```python
from build123d import *

# Parameters (mm, degrees)
SKETCH1_W                = 18
SKETCH1_H                = 10
BOSS_EXTRUDE1_DEPTH      = 10
SKETCH2_W                = 3
SKETCH2_H                = 5.5
BOSS_EXTRUDE2_DEPTH      = 4
SKETCH3_W                = 3
SKETCH3_H                = 5.5
BOSS_EXTRUDE3_DEPTH      = 4
F_4_0_4_DIAMETER_HOLE1_D = 4


with BuildPart() as part:
    # Sketch1 → Boss-Extrude1 (new body)
    with BuildSketch(Plane.XZ.offset(5)):
        with Locations((-1.5, 5)):
            Rectangle(SKETCH1_W, SKETCH1_H)
    extrude(amount=-BOSS_EXTRUDE1_DEPTH)

    # Sketch2 → Boss-Extrude2 (add)
    with BuildSketch(Plane(origin=(0, 5, 0), x_dir=(-1, 0, 0), z_dir=(0, 1, 0))):
        with Locations((-6, 2.75)):
            Rectangle(SKETCH2_W, SKETCH2_H)
    extrude(amount=BOSS_EXTRUDE2_DEPTH)

    # Sketch3 → Boss-Extrude3 (add)
    with BuildSketch(Plane.XZ.offset(5)):
        with Locations((6, 2.75)):
            Rectangle(SKETCH3_W, SKETCH3_H)
    extrude(amount=BOSS_EXTRUDE3_DEPTH)

    # Sketch4 → Cut-Revolve1 (revolve, cut)
    with BuildSketch(Plane.XY.offset(2.75)):
        Polygon((4.5, 7.2835), (4.5, 6.5), (7.5, 6.5), (7.5, 7.2835), (5.5, 7.2835), align=None)
    revolve(axis=Axis((4.5, 6.5, 2.75), (1, 0, 0)), mode=Mode.SUBTRACT)

    # Sketch5 → Cut-Revolve2 (revolve, cut)
    with BuildSketch(Plane.XY.offset(2.75), mode=Mode.PRIVATE) as cut_revolve2_sk:
        Polygon((4.5, -5.7165), (4.5, -6.5), (7.5, -6.5), (7.5, -5.7165), (5.5, -5.7165), align=None)
    revolve(cut_revolve2_sk.sketch.rotate(Axis((4.5, -6.5, 2.75), (1, 0, 0)), 270), axis=Axis((4.5, -6.5, 2.75), (1, 0, 0)), mode=Mode.SUBTRACT)

    # Sketch6 → Cut-Revolve3 (revolve, cut)
    with BuildSketch(Plane(origin=(0, 0, 0), x_dir=(1, 0, 0), z_dir=(0, 1, 0))):
        Polygon((4.7295, 0), (3.5, 0), (3.5, -10), (4.7295, -10), (4.7295, -8), align=None)
    revolve(axis=Axis((3.5, 0, 0), (0, 0, 1)), mode=Mode.SUBTRACT)

    # Ø4.0 (4) Diameter Hole1 (through all)
    with Locations(Plane(origin=(0, 0, 0), x_dir=(-1, 0, 0), z_dir=(0, 0, -1))):
        with Locations((6.5, 0)):
            Hole(F_4_0_4_DIAMETER_HOLE1_D / 2)


solid = part.part
```
Design review of the part built by this model. Coordinates are the model's own, in mm. A direction names the side the tool comes from. Give positions to 0.01 mm unless a question says otherwise; leave off trailing zeros. Loops run counter-clockwise (first coordinate to the right, second up) from the corner with the lowest first, then second, coordinate; pieces in that order, holes last. Notation, with made-up numbers: M 41.5,-21 L 52.5,-21 A33 ccw 52.5,8 Z; hole C 65.5,-20.5 d11. An arc over 180 degrees is marked long. Return JSON: item names as keys, results as strings. Group by question number.
Item 1: We need section A-A (z = 2.75). Give the boundary of the cut face in (x, y), and give its area (3 significant figures).
Item 2: We need section D-D (z = 4). Give the boundary of the cut face in (x, y).
Item 3: Insertion check: pin 1 Ø3 at (y, z) = (8, 4) entering from -X; pin 2 Ø0.9 at (x, y) = (6, -8) entering from +Z; pin 3 Ø2 at (x, z) = (3.5, 8.5) entering from +Y. Each pin has a flat end and moves straight along its axis. Give the tip position at first contact, or say it passes through.
Item 4: For probe 1 along Y at (x, z) = (5, 2.5); probe 2 along X at (y, z) = (-0.75, 8.5); probe 3 along Z at (x, y) = (6.75, 6.5), list the stretches that pass through material, from the lowest coordinate up.
Item 5: We need section B-B (y = -6.5). Give the boundary of the cut face in (x, z).
Item 6: We need section C-C (x = 3.5). Give the boundary of the cut face in (y, z).
Item 7: Mouldability with a two-part tool opening along Y and no side actions: class faces 5 (the flat face through (6, 9, 3)), 6 (the cylindrical face through (-8.1, -1.2, 5.1)), 7 (the flat face through (6, -7, 5.5)) as released by +Y, released by -Y, zero draft, split by the parting line, or undercut.
Item 8: Tool access review of faces 1 (the flat face through (4.5, -7.4, 2.1)), 2 (the flat face through (-2, 0, 10)), 3 (the flat face through (4.5, 7.4, 2.1)), 4 (the flat face through (6, 7, 5.5)): name each direction out of +Z, -Z, +X, -X, +Y, -Y from which nothing blocks a thin tool from reaching the whole face with its end or side.
Output:
{
 "1": {"outline": "M -10.5,-5 L 4.5,-5 L 4.5,-5.72 L 7.5,-5.72 L 7.5,5.72 L 4.5,5.72 L 4.5,5 L -10.5,5 Z; M 4.5,-9 L 7.5,-9 L 7.5,-7.28 L 4.5,-7.28 Z; M 4.5,7.28 L 7.5,7.28 L 7.5,9 L 4.5,9 Z; hole C -6.5,0 d4; hole C 3.5,0 d2.46", "area": "177 mm^2"},
 "2": {"outline": "M -10.5,-5 L 4.5,-5 L 4.5,-9 L 7.5,-9 L 7.5,9 L 4.5,9 L 4.5,5 L -10.5,5 Z; hole C -6.5,0 d4; hole C 3.5,0 d2.46"},
 "3": {"pin 1": "stops at x = 4.5", "pin 2": "stops at z = 5.5", "pin 3": "stops at y = 5"},
 "4": {"probe 1": "y = -9 to -7.24, -5.76 to 5.76, 7.24 to 9", "probe 2": "x = -10.5 to -8.35, -4.65 to 2.53, 4.47 to 7.5", "probe 3": "z = 0 to 1.97, 3.53 to 5.5"},
 "5": {"outline": "M 4.5,0 L 7.5,0 L 7.5,1.97 L 4.5,1.97 Z; M 4.5,3.53 L 7.5,3.53 L 7.5,5.5 L 4.5,5.5 Z"},
 "6": {"outline": "M -5,0 L -1.23,0 L -1.23,10 L -5,10 Z; M 1.23,0 L 5,0 L 5,10 L 1.23,10 Z"},
 "7": {"face 5": "released by +Y", "face 6": "undercut", "face 7": "zero draft"},
 "8": {"face 1": "+Z, -Z, -X, -Y", "face 2": "+Z, +X, -X, +Y, -Y", "face 3": "+Z, -Z, -X, +Y", "face 4": "+Z, +X, -X, +Y"}
}
